Can you work these out from the model? Positions are in its coordinate system, mm. Face numbers are marked on the shaded views. A direction names the side the tool comes from. Give positions to 0.01 mm unless a question says otherwise; leave off trailing zeros. Loops run counter-clockwise (first coordinate to the right, second up) from the corner with the lowest first, then second, coordinate; pieces in that order, holes last. Notation, with made-up numbers: (10.25, 4) - (24.25, 4) arc R8 cw to (24.25, 8) - close; hole circle Ø11 at (5, 58.25). An arc over 180 degrees is marked (long way). Use a Markdown table: item, result. Add a question column.
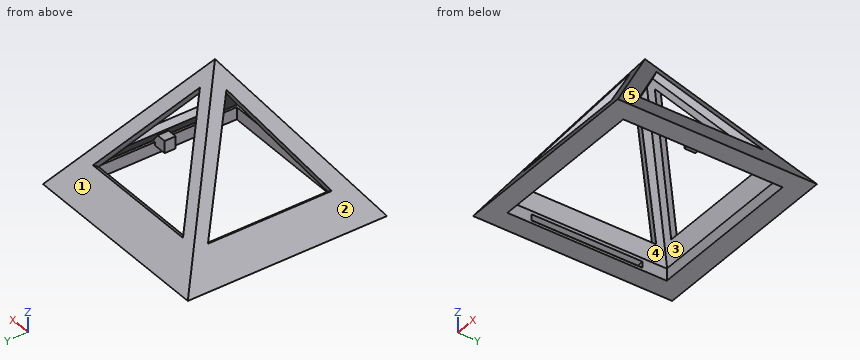
```python
from build123d import *

# Parameters (mm, degrees)
F2_W           = 90
F2_H           = 90
F6_W           = 82
F6_H           = 82
F12_DEPTH      = 5
F13_DEPTH      = 10.1
F14_DEPTH      = 10
F15_DEPTH      = 10
F17_W          = 82
F17_H          = 82
F17_W_2        = 72
F17_H_2        = 72
F18_DEPTH      = 5.5
F20_DEPTH      = 25
F20_DEPTH_BACK = 25
F21_W          = 7
F21_H          = 5
F22_DEPTH      = 4
F22_DEPTH_BACK = 1.5


with BuildPart() as f3:
    # F2 (on Top) → F3 section 0
    with BuildSketch(Plane.XY, mode=Mode.PRIVATE) as f3_s0:
        Rectangle(F2_W, F2_H)
    loft([f3_s0.sketch, Vertex(0, 0, 63.6368)])

    # F6 (on face) → F7 section 0
    with BuildSketch(Plane.XY, mode=Mode.PRIVATE) as f7_s0:
        Rectangle(F6_W, F6_H)
    loft([f7_s0.sketch, Vertex(0, 0, 58.6368)], mode=Mode.SUBTRACT)

    # F8 (on face) → F12 (cut, symmetric)
    with BuildSketch(Plane(origin=(29.9991167733, 0, 21.2135156827), x_dir=(0, 1, 0), z_dir=(0.8164845616, 0, 0.5773672666))):
        Polygon((0.1463476627, 39.9593571873), (-28.0024763197, -8.9000007138), (27.9615262598, -8.9000007138), align=None)
    extrude(amount=F12_DEPTH, both=True, mode=Mode.SUBTRACT)

    # F9 (on face) → F13 (cut)
    with BuildSketch(Plane(origin=(0, 29.9991167733, 21.2135156827), x_dir=(-1, 0, 0), z_dir=(0, 0.8164845616, 0.5773672666))):
        Polygon((0.1463476627, 39.9593571873), (-27.835653627, -8.5054690465), (28.1283489525, -8.5054690465), align=None)
    extrude(amount=-F13_DEPTH, mode=Mode.SUBTRACT)

    # F10 (on face) → F14 (cut)
    with BuildSketch(Plane(origin=(-29.9991167733, 0, 21.2135156827), x_dir=(0, -1, 0), z_dir=(-0.8164845616, 0, 0.5773672666))):
        Polygon((0.1463476627, 39.9593571873), (-28.9770383388, -9.5114903525), (26.9869642407, -9.5114903525), align=None)
    extrude(amount=-F14_DEPTH, mode=Mode.SUBTRACT)

    # F11 (on face) → F15 (cut)
    with BuildSketch(Plane(origin=(0, -29.9991167733, 21.2135156827), x_dir=(1, 0, 0), z_dir=(0, -0.8164845616, 0.5773672666))):
        Polygon((0.1463476627, 39.9593571873), (-28.0361250043, -9.3999961391), (27.9278775752, -9.3999961391), align=None)
    extrude(amount=-F15_DEPTH, mode=Mode.SUBTRACT)

    # F17 (on face) → F18 (join)
    with BuildSketch(Plane(origin=(0, 0, 0), x_dir=(1, 0, 0), z_dir=(0, 0, -1))):
        Rectangle(F17_W, F17_H)
        Rectangle(F17_W_2, F17_H_2, mode=Mode.SUBTRACT)
    extrude(amount=-F18_DEPTH)

    # F19 (on Front) → F20 (cut, two sides)
    with BuildSketch(Plane.XZ) as f20_sk:
        Polygon((-40.0405423343, 3.5011546063), (-40.0405423343, 2.0011546063), (-37.3253502548, 2.0011546063), (-36, 2.0011546063), (-36, 4.0000034512), align=None)
        with BuildLine():
            Line((-36, 2.0011546063), (-37.3253502548, 2.0011546063))
            add(Edge.make_bspline(
                [(-36, 1.16889), (-36.1044551713, 1.344294706), (-36.4561719625, 1.7902625565), (-36.9847986044, 1.9009668548), (-37.3253502548, 2.0011546063)],
                knots=[0, 0, 0, 0, 0.4677482512, 1, 1, 1, 1], degree=3))
            Line((-36, 1.16889), (-36, 2.0011546063))
        make_face()
    extrude(amount=-F20_DEPTH, mode=Mode.SUBTRACT)
    extrude(f20_sk.sketch, amount=F20_DEPTH_BACK, mode=Mode.SUBTRACT)

    # F21 (on face) → F22 (join, two sides)
    with BuildSketch(Plane.XY.offset(5.5)) as f22_sk:
        with Locations((33.4785108268, -1.5248925798)):
            Rectangle(F21_W, F21_H)
    extrude(amount=F22_DEPTH)
    extrude(f22_sk.sketch, amount=-F22_DEPTH_BACK)


solid = f3.part
```
1. Suppose I cut it at A-A (x = -31.5). List the corners of the cut face in (y, z) for me.
2. On a 3-axis mill with a long thin cutter (end or side, diameter ignored), from which of +Z, -Z, +X, -X, +Y, -Y can I reach the whole of each face in a straight line? I mean the marked faces 4 and 5. Say none if no direction works.
3. If we mould it in two halves opening along Y, with no side actions, what happens to the marked faces 1, 2 and 3? For each: released by +Y, released by -Y, zero draft, split by the parting line, or undercut.
4. Suppose I cut it at C-C (y = -31). List the corners of the cut face in (x, z) for me.
5. Please list where these lines run through material, in increasing order: line 1 along Y through (x, z) = (19, 28.5); line 2 along Z through (x, y) = (-23, -36.5); line 3 along Y through (x, z) = (13.5, 38.5). Write a range as [from, to].
6. Suppose I cut it at B-B (z = 37). List the corners of the cut face in (x, y) for me.
7. Suppose I cut it at D-D (x = -17.5). List the corners of the cut face in (y, z) for me.
8. Will these pins go through, and if not, where does the flat tip stop? P1, Ø0.8, axis at y = 8, z = 2.5, coming from the +X side (3 decimals); P2, Ø2.5, axis at y = -1.5, z = 6, coming from the -X side; P3, Ø1, axis at x = 13, y = 8.5, coming from the -Z side.
Results below:
| question | item | result |
|---|---|---|
| 1 | outline | (-45, 0) - (-36, 0) - (-36, 5.5) - (-37.15, 5.5) - (-31.5, 13.59) - (-25.68, 13.59) - (-23.24, 19.09) - (-31.5, 19.09) - close; (24.91, 19.09) - (27.55, 13.59) - (31.5, 13.59) - (37.15, 5.5) - (36, 5.5) - (36, 0) - (45, 0) - (31.5, 19.09) - close |
| 2 | face 4 | none |
| 2 | face 5 | +Z, +X, +Y, -Y |
| 3 | face 1 | released by +Y |
| 3 | face 2 | zero draft |
| 3 | face 3 | undercut |
| 4 | outline | (-45, 0) - (-36, 0) - (-36, 5.5) - (-37.15, 5.5) - (-31, 14.3) - (-26.22, 14.3) - (-23.66, 19.8) - (-31, 19.8) - close; (23.61, 19.8) - (26.14, 14.3) - (31, 14.3) - (37.15, 5.5) - (36, 5.5) - (36, 0) - (45, 0) - (31, 19.8) - close |
| 5 | line 1 | [-24.85, -21.07], [21.07, 24.85] |
| 5 | line 2 | [0, 5.5], [6.44, 12.02] |
| 5 | line 3 | [-17.78, -14.08], [14.08, 17.78] |
| 6 | outline | (-18.84, -18.84) - (-11.63, -18.84) - (-10.41, -15.13) - (-15.13, -15.13) - (-15.13, -10.18) - (-18.84, -11.34) - close; (-18.84, 12) - (-15.13, 10.74) - (-15.13, 15.13) - (-10.82, 15.13) - (-12.05, 18.84) - (-18.84, 18.84) - close; (10.53, 15.13) - (15.13, 15.13) - (15.13, 10.67) - (18.84, 11.89) - (18.84, 18.84) - (11.76, 18.84) - close; (10.55, -15.13) - (11.75, -18.84) - (18.84, -18.84) - (18.84, -11.74) - (15.13, -10.5) - (15.13, -15.13) - close |
| 7 | outline | (-45, 0) - (-36, 0) - (-36, 5.5) - (-37.15, 5.5) - (-32.82, 11.7) - (-35.43, 13.54) - close; (-24.77, 28.61) - (-22.25, 26.82) - (-17.5, 33.61) - (-12.42, 33.61) - (-10.08, 38.89) - (-17.5, 38.89) - close; (10.63, 38.89) - (13.17, 33.61) - (17.5, 33.61) - (21.76, 27.52) - (24.28, 29.3) - (17.5, 38.89) - close; (32.31, 12.43) - (37.15, 5.5) - (36, 5.5) - (36, 0) - (45, 0) - (34.91, 14.27) - close |
| 8 | P1 | x = 43.515 |
| 8 | P2 | x = -41.64 |
| 8 | P3 | z = 39.58 |
